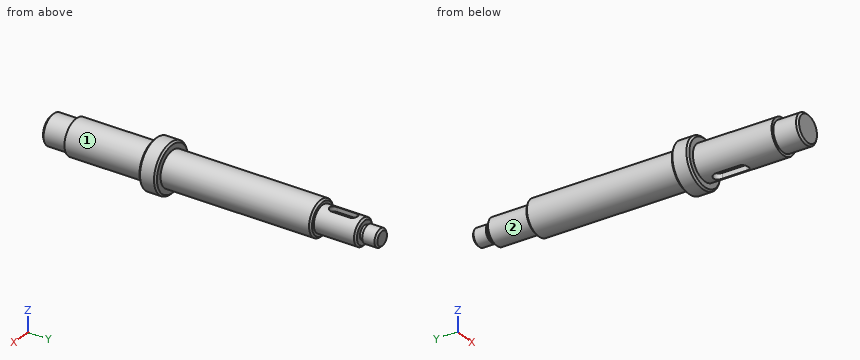
```python
from build123d import *

# Parameters (mm, degrees)
CHAMFER1_SIZE      = 1
CUT_EXTRUDE1_DEPTH = 3
CUT_EXTRUDE2_DEPTH = 3.5


with BuildPart() as part:
    # Sketch1 → Revolve1 (revolve)
    with BuildSketch(Plane.XY, mode=Mode.PRIVATE) as revolve1_sk:
        Polygon((0, 0), (0, -189), (-8.5, -189), (-8.5, -175), (-10, -175), (-10, -130), (-14, -130), (-14, -120), (-10, -120), (-10, -34), (-7.5, -34), (-7.5, -10), (-4, -10), (-4, -8), (-5, -8), (-5, 0), align=None)
    revolve(revolve1_sk.sketch.rotate(Axis((0, 0, 0), (0, -1, 0)), 270), axis=Axis((0, 0, 0), (0, -1, 0)))

    # Chamfer1
    chamfer1_edges = [part.edges().sort_by_distance(p)[0] for p in [
        (0, -189, -8.5),
        (0, -130, -14),
        (0, -120, -14),
        (0, -34, -10),
        (0, -10, -7.5),
        (0, 0, -5),
    ]]
    chamfer(chamfer1_edges, length=CHAMFER1_SIZE)

    # Sketch2 → Cut-Extrude1 (cut)
    with BuildSketch(Plane.XY.offset(7.5)):
        with BuildLine():
            Line((2.5, -16.5), (2.5, -27.5))
            ThreePointArc((2.5, -27.5), (0, -30), (-2.5, -27.5))
            Line((-2.5, -27.5), (-2.5, -16.5))
            ThreePointArc((-2.5, -16.5), (0, -14), (2.5, -16.5))
        make_face()
    extrude(amount=-CUT_EXTRUDE1_DEPTH, mode=Mode.SUBTRACT)

    # Sketch3 → Cut-Extrude2 (cut)
    with BuildSketch(Plane.XY.offset(-10)):
        with BuildLine():
            Line((-3, -152), (-3, -138))
            ThreePointArc((-3, -138), (0, -135), (3, -138))
            Line((3, -138), (3, -152))
            ThreePointArc((3, -152), (0, -155), (-3, -152))
        make_face()
    extrude(amount=CUT_EXTRUDE2_DEPTH, mode=Mode.SUBTRACT)


solid = part.part
```
Model file for the job. Use its own axes, mm. Face numbers are marked on the shaded views. A direction names the side the tool comes from. Round coordinates to 2 decimals unless told otherwise and drop trailing zeros. Order: outer loops, then holes, each group sorted by start corner. A loop starts at its lowest first (then second) coordinate and runs counter-clockwise, first axis right, second up. Notation, with made-up numbers: M 35.5,-31 L 48.5,-31 A17 ccw 48.5,-10 Z; hole C -0.5,-2 d5. An arc over 180 degrees is marked long. Use CSV: the item, a comma, the result in double quotes.
Item 1: Saw through at A-A (y = -148.5). List the corners of the cut face in (x, z), plus the area to 3 significant figures.
Worked answers:
outline,"M -3,-9.54 L -3,-6.5 L 3,-6.5 L 3,-9.54 A10 ccw long Z"
area,"294 mm²"
Item 2: Which spindle directions (+Z, -Z, +X, -X, +Y, -Y) get a long thin tool onto all of the face, cutting with end or side? Do the marked faces 1 and 2. Say none if no direction does.
Worked answers:
face 1,"-Y"
face 2,"+Y"
Item 3: Pin check, flat tips, straight feed: pin 1 (6 mm diameter, centred on x = 8, y = -95, fed in from -Z); pin 2 (3 mm diameter, centred on y = -68, z = -2, fed in from -X); pin 3 (2 mm diameter, centred on y = -23.5, z = 6, fed in from -X); pin 4 (1 mm diameter, centred on y = -80.5, z = 11, fed in from -X). Stop position of each tip, or through.
Worked answers:
pin 1,"z = -8.66"
pin 2,"x = -9.99"
pin 3,"x = -5.59"
pin 4,"through"
Item 4: Saw through at B-B (y = -168). List the corners of the cut face in (x, z), plus the area to 3 significant figures.
Worked answers:
outline,"C 0,0 d20"
area,"314 mm²"
Item 5: Probe probe 1 along Y at (x, z) = (-8, 10.25); probe 2 along Y at (x, z) = (-3, 8); probe 3 along Y at (x, z) = (2, -8). List the from-to ranges inside material, lowest first.
Worked answers:
probe 1,"-130 to -120"
probe 2,"-175 to -34"
probe 3,"-188.25 to -154.24, -135.76 to -34"
